```python
from build123d import *

# Parameters (mm, degrees)
SKETCH1_W                                           = 158
SKETCH1_H                                           = 124
BOSS_EXTRUDE1_DEPTH                                 = 5.9
CSK_FOR_M3_FLAT_HEAD_MACHINE_SCREW1_D               = 3.4
CSK_FOR_M3_FLAT_HEAD_MACHINE_SCREW1_DEPTH           = 10
CSK_FOR_M3_FLAT_HEAD_MACHINE_SCREW1_CSINK_D         = 6.3
CSK_FOR_M3_FLAT_HEAD_MACHINE_SCREW1_CSINK_ANGLE     = 90
CSK_FOR_M3_FLAT_HEAD_MACHINE_SCREW1_TIP             = 1.021463052
CSK_FOR_1_4_FLAT_HEAD_MACHINE_SCREW_100_D           = 7.14248
CSK_FOR_1_4_FLAT_HEAD_MACHINE_SCREW_100_CSINK_D     = 12.8778
CSK_FOR_1_4_FLAT_HEAD_MACHINE_SCREW_100_CSINK_ANGLE = 100


with BuildPart() as part:
    # Sketch1 → Boss-Extrude1 (new body)
    with BuildSketch(Plane.XY):
        Rectangle(SKETCH1_W, SKETCH1_H)
    extrude(amount=BOSS_EXTRUDE1_DEPTH)

    # CSK for M3 Flat Head Machine Screw1
    with Locations(Plane.XY.offset(5.9)):
        with Locations((-67.1, 56), (67.1, 56)):
            CounterSinkHole(CSK_FOR_M3_FLAT_HEAD_MACHINE_SCREW1_D / 2, CSK_FOR_M3_FLAT_HEAD_MACHINE_SCREW1_CSINK_D / 2, depth=CSK_FOR_M3_FLAT_HEAD_MACHINE_SCREW1_DEPTH, counter_sink_angle=CSK_FOR_M3_FLAT_HEAD_MACHINE_SCREW1_CSINK_ANGLE)
            with Locations((0, 0, -(CSK_FOR_M3_FLAT_HEAD_MACHINE_SCREW1_DEPTH + CSK_FOR_M3_FLAT_HEAD_MACHINE_SCREW1_TIP / 2))):  # 118° drill point
                Cone(0, CSK_FOR_M3_FLAT_HEAD_MACHINE_SCREW1_D / 2, CSK_FOR_M3_FLAT_HEAD_MACHINE_SCREW1_TIP, mode=Mode.SUBTRACT)

    # CSK for 1/4 Flat Head Machine Screw (100)1 (through all)
    with Locations(Plane(origin=(0, 0, 0), x_dir=(1, 0, 0), z_dir=(0, 0, -1))):
        with Locations((-17.81875, -44.268219257), (17.81875, -44.268219257)):
            CounterSinkHole(CSK_FOR_1_4_FLAT_HEAD_MACHINE_SCREW_100_D / 2, CSK_FOR_1_4_FLAT_HEAD_MACHINE_SCREW_100_CSINK_D / 2, counter_sink_angle=CSK_FOR_1_4_FLAT_HEAD_MACHINE_SCREW_100_CSINK_ANGLE)


solid = part.part
```
For this review, take the finished solid that the model builds, in its own axes (mm). Give positions to 0.01 mm unless a question says otherwise; leave off trailing zeros. Write each loop counter-clockwise with the first axis right and the second up, starting at its lowest first coordinate (ties: lowest second). Pieces come first, ordered by that corner, then holes.
Item 1: Take a section at A-A (x = -67.1). Give the boundary of the cut face in (y, z), and give its area (3 significant figures).
Item 2: Insertion check: P1, Ø8, axis at x = -17.82, y = 44.27, coming from the -Z side; P2, Ø5.5, axis at x = 17.82, y = 44.27, coming from the +Z side. Each pin has a flat end and moves straight along its axis. Give the tip position at first contact, or say it passes through.
Item 3: Take a section at B-B (y = 56). Give the boundary of the cut face in (x, z), and give its area (3 significant figures).
Item 4: Wall thickness on probe 1 along X at (y, z) = (56, 1.4); probe 2 along X at (y, z) = (45, 5.6); probe 3 along Y at (x, z) = (67.1, 3.55): over which ranges is each line inside the solid? List them lowest first.
Item 5: The part is to be moulded in two halves that separate along X. For faces 1 (the face through (-79, -1, 3)), 2 (the face through (-14.25, 44.11, 4.18)), 3 (the face through (-14.874, 46.526, 2.289)), 4 (the face through (79, -1, 3)), say which applies: +X half, -X half, draft (parallel to the pull), parting line (faces both ways), or undercut.
Established:
1. outline: (-62, 0) - (54.3, 0) - (54.3, 4.45) - (52.85, 5.9) - (-62, 5.9) - close; (57.7, 0) - (62, 0) - (62, 5.9) - (59.15, 5.9) - (57.7, 4.45) - close
1. area: 709 mm2
2. P1: stops at z = 2.04
2. P2: passes through
3. outline: (-79, 0) - (-68.8, 0) - (-68.8, 4.45) - (-70.25, 5.9) - (-79, 5.9) - close; (-65.4, 0) - (65.4, 0) - (65.4, 4.45) - (63.95, 5.9) - (-63.95, 5.9) - (-65.4, 4.45) - close; (68.8, 0) - (79, 0) - (79, 5.9) - (70.25, 5.9) - (68.8, 4.45) - close
3. area: 888 mm2
4. probe 1: x = -79 to -68.8, -65.4 to 65.4, 68.8 to 79
4. probe 2: x = -79 to -21.31, -14.32 to 14.32, 21.31 to 79
4. probe 3: y = -62 to 54.3, 57.7 to 62
5. face 1: -X half
5. face 2: undercut
5. face 3: undercut
5. face 4: +X half
